Design review of the part built by this model. Coordinates are the model's own, in mm. Face numbers are marked on the shaded views. A direction names the side the tool comes from. Coordinates: 2 decimals unless noted, no trailing zeros. Order: outer loops, then holes, each group sorted by start corner. A loop starts at its lowest first (then second) coordinate and runs counter-clockwise, first axis right, second up. Notation, with made-up numbers: (-2, 36) - (2, 36) arc R15 cw to (2, 44) - close; hole circle Ø5 at (-30, 57.25). An arc over 180 degrees is marked (long way). Write each question's results on one line, items separated by ' | '. Start each with the question number.
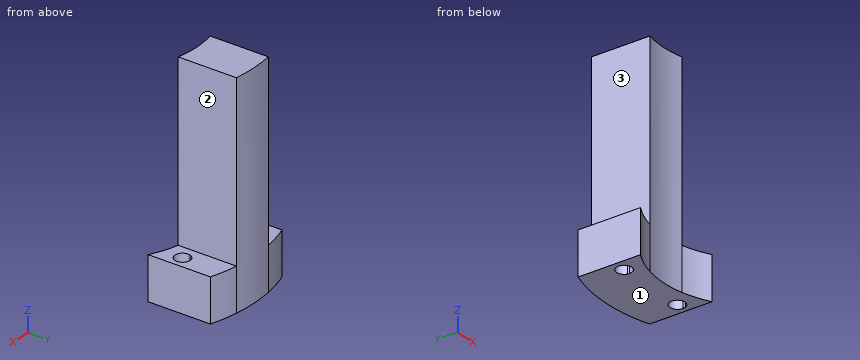
```python
from build123d import *

# Parameters (mm, degrees)
F1_DEPTH = 10
F2_DEPTH = 50


with BuildPart() as f1:
    # F0 (on Top) → F1 (new body)
    with BuildSketch(Plane.XY):
        with BuildLine():
            Line((-11.1938343047, 34.2154654149), (-11.1938343047, 24.5702680807))
            ThreePointArc((-11.1938343047, 24.5702680807), (-10.5947366889, 24.8344831735), (-9.9894082697, 25.0840930157))
            ThreePointArc((-9.9894082697, 25.0840930157), (-8.8842385883, 27.3428748435), (-6.6624588878, 26.1650843983))
            ThreePointArc((-6.6624588878, 26.1650843983), (-5.8286474975, 26.3633622353), (-4.988963041, 26.5350758012))
            Line((-4.988963041, 26.5350758012), (-4.988963041, 35.6526331114))
            ThreePointArc((-4.988963041, 35.6526331114), (-8.1232441321, 35.0715398118), (-11.1938343047, 34.2154654149))
        make_face()
        with BuildLine():
            ThreePointArc((-4.988963041, 26.5350758012), (0, 27), (4.988963041, 26.5350758012))
            Line((4.988963041, 26.5350758012), (4.988963041, 35.6526331114))
            ThreePointArc((4.988963041, 35.6526331114), (0, 36), (-4.988963041, 35.6526331114))
            Line((-4.988963041, 35.6526331114), (-4.988963041, 26.5350758012))
        make_face()
        with BuildLine():
            ThreePointArc((9.9894082697, 25.0840930157), (10.5947366889, 24.8344831735), (11.1938343047, 24.5702680807))
            Line((11.1938343047, 24.5702680807), (11.1938343047, 34.2154654149))
            ThreePointArc((11.1938343047, 34.2154654149), (8.1232441321, 35.0715398118), (4.988963041, 35.6526331114))
            Line((4.988963041, 35.6526331114), (4.988963041, 26.5350758012))
            ThreePointArc((4.988963041, 26.5350758012), (5.8286474975, 26.3633622353), (6.6624588878, 26.1650843983))
            ThreePointArc((6.6624588878, 26.1650843983), (8.5891721662, 27.4111900636), (10.0934588481, 25.67852594))
            ThreePointArc((10.0934588481, 25.67852594), (10.0672499445, 25.3767905326), (9.9894082697, 25.0840930157))
        make_face()
        with BuildLine():
            ThreePointArc((4.988963041, 22.1962327384), (8.1792145377, 21.2288235554), (11.1938343047, 19.8055692561))
            Line((11.1938343047, 19.8055692561), (11.1938343047, 24.5702680807))
            ThreePointArc((11.1938343047, 24.5702680807), (10.5947366889, 24.8344831735), (9.9894082697, 25.0840930157))
            ThreePointArc((9.9894082697, 25.0840930157), (7.802679108, 24.0141770365), (6.6624588878, 26.1650843983))
            ThreePointArc((6.6624588878, 26.1650843983), (5.8286474975, 26.3633622353), (4.988963041, 26.5350758012))
            Line((4.988963041, 26.5350758012), (4.988963041, 22.1962327384))
        make_face()
        with BuildLine():
            Line((-11.1938343047, 24.5702680807), (-11.1938343047, 19.8055692561))
            ThreePointArc((-11.1938343047, 19.8055692561), (-8.1792145377, 21.2288235554), (-4.988963041, 22.1962327384))
            Line((-4.988963041, 22.1962327384), (-4.988963041, 26.5350758012))
            ThreePointArc((-4.988963041, 26.5350758012), (-5.8286474975, 26.3633622353), (-6.6624588878, 26.1650843983))
            ThreePointArc((-6.6624588878, 26.1650843983), (-6.6107947245, 25.9242392581), (-6.5934588481, 25.67852594))
            ThreePointArc((-6.5934588481, 25.67852594), (-8.0417234407, 23.9547348436), (-9.9894082697, 25.0840930157))
            ThreePointArc((-9.9894082697, 25.0840930157), (-10.5947366889, 24.8344831735), (-11.1938343047, 24.5702680807))
        make_face()
        with BuildLine():
            ThreePointArc((-4.988963041, 22.1962327384), (0, 22.75), (4.988963041, 22.1962327384))
            Line((4.988963041, 22.1962327384), (4.988963041, 26.5350758012))
            ThreePointArc((4.988963041, 26.5350758012), (0, 27), (-4.988963041, 26.5350758012))
            Line((-4.988963041, 26.5350758012), (-4.988963041, 22.1962327384))
        make_face()
    extrude(amount=F1_DEPTH)

    # F0 (on Top) → F2 (join)
    with BuildSketch(Plane.XY):
        with BuildLine():
            ThreePointArc((-4.988963041, 26.5350758012), (0, 27), (4.988963041, 26.5350758012))
            Line((4.988963041, 26.5350758012), (4.988963041, 35.6526331114))
            ThreePointArc((4.988963041, 35.6526331114), (0, 36), (-4.988963041, 35.6526331114))
            Line((-4.988963041, 35.6526331114), (-4.988963041, 26.5350758012))
        make_face()
        with BuildLine():
            ThreePointArc((-4.988963041, 22.1962327384), (0, 22.75), (4.988963041, 22.1962327384))
            Line((4.988963041, 22.1962327384), (4.988963041, 26.5350758012))
            ThreePointArc((4.988963041, 26.5350758012), (0, 27), (-4.988963041, 26.5350758012))
            Line((-4.988963041, 26.5350758012), (-4.988963041, 22.1962327384))
        make_face()
    extrude(amount=F2_DEPTH)


solid = f1.part
```
(1) Tool access review of the marked faces 1, 2 and 3: name each direction out of +Z, -Z, +X, -X, +Y, -Y from which nothing blocks a thin tool from reaching the whole face with its end or side.
(2) Take a section at A-A (z = 5). State the section outline as (x, y) points.
(3) Take a section at C-C (x = 9). State the section outline as (y, z) points.
(4) Take a section at B-B (y = 33.5). State the section outline as (x, z) points.
(5) Take a section at D-D (z = 29.5). State the section outline as (x, y) points, plus the area to 3 significant figures.
(6) Clearance check with flat-ended pins moving along their axes: pin 1 (1 mm diameter, centred on x = -6.5, z = 5.5, fed in from +Y); pin 2 (8 mm diameter, centred on x = -8.5, z = 40, fed in from -Y); pin 3 (1 mm diameter, centred on y = 26, z = 27, fed in from -X). State where each tip first meets the part, or that it passes through.
(7) To check wall thickness, follow line 1 along X through (y, z) = (34.75, 30.5); line 2 along Z through (x, y) = (9, 22.25); line 3 along Y through (x, z) = (-0.5, 34.5). State the ranges of each line that lie inside material, in increasing order. Write a range as [from, to].
Worked out:
1) face 1: -Z, +X, -X, +Y, -Y | face 2: +Z, +X, +Y, -Y | face 3: +Z, -X, +Y, -Y
2) outline: (-11.19, 19.81) arc R22.75 cw to (11.19, 19.81) - (11.19, 34.22) arc R36 ccw to (-11.19, 34.22) - close; hole circle Ø3.5 at (-8.34, 25.68); hole circle Ø3.5 at (8.34, 25.68)
3) outline: (20.89, 0) - (24.06, 0) - (24.06, 10) - (20.89, 10) - close; (27.3, 0) - (34.86, 0) - (34.86, 10) - (27.3, 10) - close
4) outline: (-11.19, 0) - (11.19, 0) - (11.19, 10) - (4.99, 10) - (4.99, 50) - (-4.99, 50) - (-4.99, 10) - (-11.19, 10) - close
5) outline: (-4.99, 22.2) arc R22.75 cw to (4.99, 22.2) - (4.99, 35.65) arc R36 ccw to (-4.99, 35.65) - close | area: 133 mm^2
6) pin 1: y = 35.5 | pin 2: y = 22.2 | pin 3: x = -4.99
7) line 1: [-4.99, 4.99] | line 2: [0, 10] | line 3: [22.74, 36]
